Geometry check sheet. Reference: the model listing, model coordinates, mm. A direction names the side the tool comes from. Give positions to 0.01 mm unless a question says otherwise; leave off trailing zeros. Write each loop counter-clockwise with the first axis right and the second up, starting at its lowest first coordinate (ties: lowest second). Pieces come first, ordered by that corner, then holes. Notation, with made-up numbers: (53, -15) - (82, -15) arc R11 cw to (82, -11) - close; hole circle Ø8 at (85.5, -13). An arc over 180 degrees is marked (long way). Write item = value, one per line. Start each with the question number.
(1) Access from +Z, -Z, +X, -X, +Y, -Y to the whole of each face (thin tool, end or side, straight path). Record for faces 4 (the flat face through (-1, -1, 6)), 5 (the flat face through (-7.637, 0, 1)), 6 (the flat face through (-1, 1, 6)).
(2) Section check B-B, the plane x = 0. Enter the section's corners in (y, z), plus the area to 3 significant figures.
(3) Section check A-A, the plane y = 0. Enter the section's corners in (x, z).
(4) Depth check by flat-ended pin: pin 1 Ø1.5 at (x, y) = (4.5, 1) entering from +Z; pin 2 Ø1.5 at (y, z) = (1, 6) entering from -X. Enter the tip coordinate at first touch or a pass-through.
(5) Section check D-D, the plane y = 1.25. Enter the section's corners in (x, z), plus the area to 3 significant figures.
(6) Thickness scan on L1, parallel to Z at x = 0, y = 0.1; L2, parallel to Z at x = -3.5, y = 2; L3, parallel to Y at x = 2, z = 6.75. Record the ranges inside material, lowest first.
(7) Draft check along X on faces 1 (the cylindrical face through (13.089, -0.766, 0.986)), 2 (the cylindrical face through (0.039, -0.014, 7.753)), 3 (the flat face through (4, -3.873, 1)). Enter one of: pulls with the +X half, pulls with the -X half, needs draft (parallel to the pull), parting line crosses it, or undercut.
(8) Section check C-C, the plane z = 3.5. Enter the section's corners in (x, y), plus the area to 3 significant figures.
```python
from build123d import *

# Parameters (mm, degrees)
F0_W     = 23.9590460792
F0_H     = 7.6507304548
F0_R     = 2
F1_DEPTH = 2
F2_R     = 1.75
F3_DEPTH = 1


# Not quite as in the source:
# - a feature names something its author has since deleted; it is built from what else it names


with BuildPart() as f1:
    # F0 (on Top) → F1 (new body)
    with BuildSketch(Plane.XY):
        with Locations((4.3424949229, -0.0471555286)):
            Rectangle(F0_W, F0_H)
        with Locations((11.2411081956, 0)):
            Circle(F0_R, mode=Mode.SUBTRACT)
    extrude(amount=F1_DEPTH)

    # F2 (on Front) → F3 (join, symmetric)
    with BuildSketch(Plane.XZ):
        with BuildLine():
            Line((-2.4094440999, 6.5410234491), (-5.7779996579, 2))
            Line((-5.7779996579, 2), (5.7779996579, 2))
            Line((5.7779996579, 2), (2.4094440999, 6.5410234491))
            ThreePointArc((2.4094440999, 6.5410234491), (0, 7.7536848887), (-2.4094440999, 6.5410234491))
        make_face()
        with Locations((0, 4.3635135517)):
            Circle(F2_R, mode=Mode.SUBTRACT)
    extrude(amount=F3_DEPTH, both=True)


solid = f1.part
```
Model answer:
q1.face_4 = +Z, +X, -X, -Y
q1.face_5 = +Z, -Z, -X, +Y, -Y
q1.face_6 = +Z, +X, -X, +Y
q2.outline = (-3.87, 0) - (3.78, 0) - (3.78, 2) - (1, 2) - (1, 2.61) - (-1, 2.61) - (-1, 2) - (-3.87, 2) - close; (-1, 6.11) - (1, 6.11) - (1, 7.75) - (-1, 7.75) - close
q2.area = 19.8 mm²
q3.outline = (-7.64, 0) - (9.24, 0) - (9.24, 2) - (5.78, 2) - (2.41, 6.54) arc R3 ccw to (-2.41, 6.54) - (-5.78, 2) - (-7.64, 2) - close; (13.24, 0) - (16.32, 0) - (16.32, 2) - (13.24, 2) - close; hole circle Ø3.5 at (0, 4.36)
q4.pin_1 = 4.73
q4.pin_2 = -3.37
q5.outline = (-7.64, 0) - (9.68, 0) - (9.68, 2) - (-7.64, 2) - close; (12.8, 0) - (16.32, 0) - (16.32, 2) - (12.8, 2) - close
q5.area = 41.7 mm²
q6.L1 = 0 to 2.61, 6.11 to 7.75
q6.L2 = 0 to 2
q6.L3 = -1 to 1
q7.face_1 = undercut
q7.face_2 = parting line crosses it
q7.face_3 = needs draft
q8.outline = (-4.67, -1) - (-1.52, -1) - (-1.52, 1) - (-4.67, 1) - close; (1.52, -1) - (4.67, -1) - (4.67, 1) - (1.52, 1) - close
q8.area = 12.6 mm²
